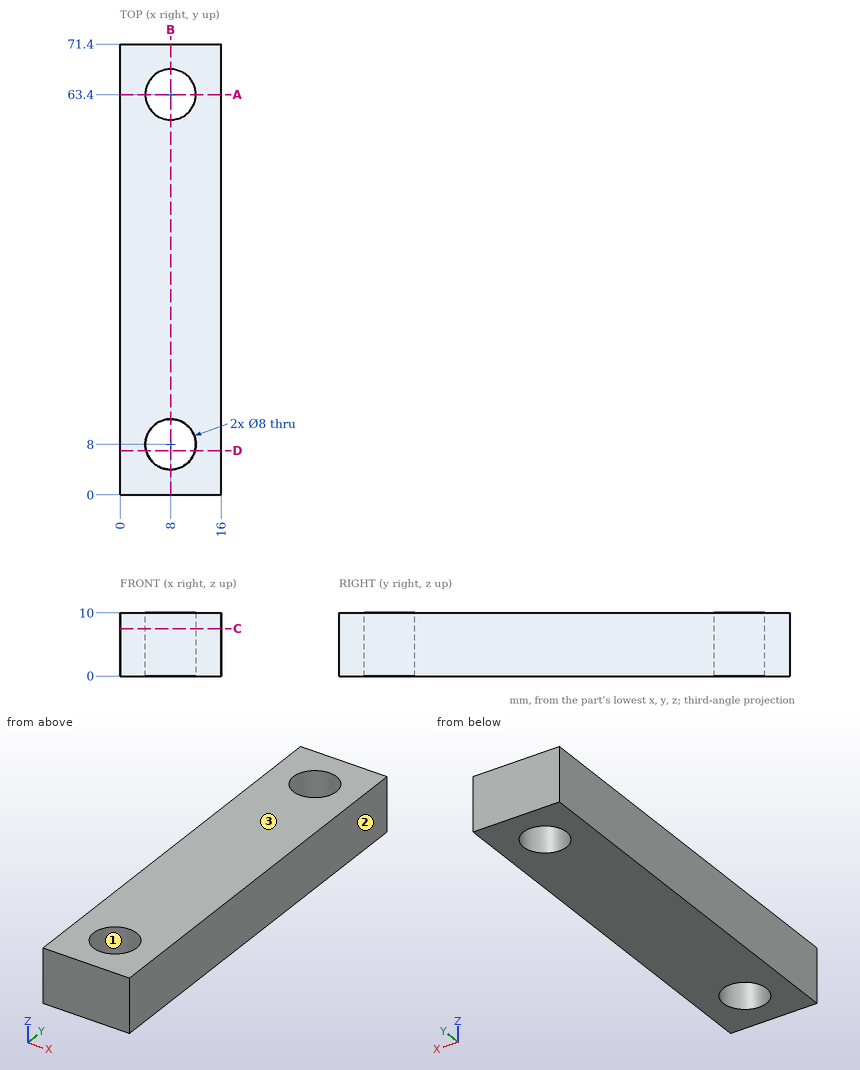
Could you check a few things on this drawing? It's one solid part, dimensions in mm from its lowest x, y, z. Give positions to 0.01 mm unless a question says otherwise; leave off trailing zeros. Write each loop counter-clockwise with the first axis right and the second up, starting at its lowest first coordinate (ties: lowest second). Pieces come first, ordered by that corner, then holes. Notation, with made-up numbers: (21.25, 43) -> (67.25, 43) arc R24 cw to (67.25, 56) -> close; hole circle Ø5 at (-27.5, 16). An arc over 180 degrees is marked (long way). Write each question's results on one line, items separated by ' | '.
1. I want a section at C-C, the plane z = 7.5. Write out the boundary of the cut face in (x, y).
Check sheet entries:
outline: (0, 0) -> (16, 0) -> (16, 71.4) -> (0, 71.4) -> close; hole circle Ø8 at (8, 8); hole circle Ø8 at (8, 63.4)
2. If we mould it in two halves opening along X, with no side actions, what happens to the marked faces 1, 2 and 3? For each: released by +X, released by -X, zero draft, split by the parting line, or undercut.
Check sheet entries:
face 1: undercut | face 2: released by +X | face 3: zero draft
3. Will this pin go through, and if not, where does the flat tip stop? pin 1 Ø4 at (x, y) = (10.5, 58) entering from -Z.
Check sheet entries:
pin 1: stops at z = 0
4. I want a section at D-D, the plane y = 7. Write out the boundary of the cut face in (x, z).
Check sheet entries:
outline: (0, 0) -> (4.13, 0) -> (4.13, 10) -> (0, 10) -> close; (11.87, 0) -> (16, 0) -> (16, 10) -> (11.87, 10) -> close
5. I want a section at B-B, the plane x = 8. Write out the boundary of the cut face in (y, z).
Check sheet entries:
outline: (0, 0) -> (4, 0) -> (4, 10) -> (0, 10) -> close; (12, 0) -> (59.4, 0) -> (59.4, 10) -> (12, 10) -> close; (67.4, 0) -> (71.4, 0) -> (71.4, 10) -> (67.4, 10) -> close
6. I need wall thicknesses on L1, parallel to Y at x = 8, z = 3.75; L2, parallel to Y at x = 4.5, z = 8.25; L3, parallel to X at y = 4.5, z = 1.5. Which ranges of each line are inside material? Lowest first, please.
Check sheet entries:
L1: y = 0 to 4, 12 to 59.4, 67.4 to 71.4 | L2: y = 0 to 6.06, 9.94 to 61.46, 65.34 to 71.4 | L3: x = 0 to 6.06, 9.94 to 16
7. I want a section at A-A, the plane y = 63.4. Write out the boundary of the cut face in (x, z).
Check sheet entries:
outline: (0, 0) -> (4, 0) -> (4, 10) -> (0, 10) -> close; (12, 0) -> (16, 0) -> (16, 10) -> (12, 10) -> close
